Model file for the job. Use its own axes, mm. Face numbers are marked on the shaded views. Give positions to 0.01 mm unless a question says otherwise; leave off trailing zeros. Write each loop counter-clockwise with the first axis right and the second up, starting at its lowest first coordinate (ties: lowest second). Pieces come first, ordered by that corner, then holes.
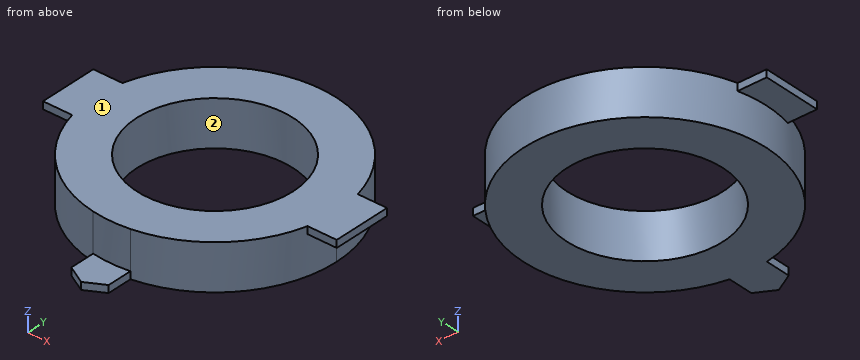
```python
from build123d import *

# Parameters (mm, degrees)
F1_DEPTH = 6.24
F2_DEPTH = 1
F3_R     = 10.71
F4_DEPTH = 6.241
F6_DEPTH = 1


# Not quite as in the source:
# - a pattern or mirror of a feature is missing from the dataset's text; its kind, count and spacing are read off the source's solid


with BuildPart() as f1:
    # F0 (on Top) → F1 (new body)
    with BuildSketch(Plane.XY):
        with BuildLine():
            ThreePointArc((2.56, -16.4317771407), (12.6318981155, -10.8162863313), (16.63, 0))
            ThreePointArc((16.63, 0), (-10.8162863313, 12.6318981155), (-2.56, -16.4317771407))
            ThreePointArc((-2.56, -16.4317771407), (0, -16.63), (2.56, -16.4317771407))
        make_face()
    extrude(amount=F1_DEPTH)

    # F0 (on Top) → F2 (join)
    with BuildSketch(Plane.XY):
        with BuildLine():
            ThreePointArc((2.56, -16.4317771407), (0, -16.63), (-2.56, -16.4317771407))
            Line((-2.56, -16.4317771407), (-2.56, -19.8917771407))
            Line((-2.56, -19.8917771407), (0, -21.31))
            Line((0, -21.31), (2.56, -19.8917771407))
            Line((2.56, -19.8917771407), (2.56, -16.4317771407))
        make_face()
    extrude(amount=F2_DEPTH)

    # F3 (on face) → F4 (cut, through all)
    with BuildSketch(Plane.XY.offset(6.24)):
        Circle(F3_R)
    extrude(amount=-F4_DEPTH, mode=Mode.SUBTRACT)

    # F5 (on face) → F6 (join)
    with BuildSketch(Plane.XY.offset(6.24)):
        with BuildLine():
            Line((20.1417749953, 4), (16.1417749953, 4))
            ThreePointArc((16.1417749953, 4), (16.5074925136, 2.0148426524), (16.63, 0))
            ThreePointArc((16.63, 0), (16.5074925136, -2.0148426524), (16.1417749953, -4))
            Line((16.1417749953, -4), (20.1417749953, -4))
            Line((20.1417749953, -4), (20.1417749953, 4))
        make_face()
    f6 = extrude(amount=-F6_DEPTH)

    # F6_copies: F6 across plane
    add(f6.mirror(Plane(origin=(0, 0, 0), x_dir=(0, 0, -1), z_dir=(-1, 0, 0))))


solid = f1.part
```
1. Slice it at D-D, the plane z = 3. Write the cut outline in (x, y), and give its area (3 significant figures).
Calculated:
outline: circle Ø33.26 at (0, 0); hole circle Ø21.42 at (0, 0)
area: 508 mm2
2. Pin check, flat tips, straight feed: P1, Ø1.2, axis at x = 18, y = -1, coming from the -Z side; P2, Ø0.5, axis at x = -17.5, z = 5.5, coming from the -Y side; P3, Ø1.1, axis at x = 18.5, z = 5.5, coming from the +Y side. Stop position of each tip, or through.
Calculated:
P1: stops at z = 5.24
P2: stops at y = -4
P3: stops at y = 4
3. Probe probe 1 along Y at (x, z) = (0, 4.5); probe 2 along X at (y, z) = (-7, 2.5); probe 3 along X at (y, z) = (3, 2). List the from-to ranges inside material, lowest first.
Calculated:
probe 1: y = -16.63 to -10.71, 10.71 to 16.63
probe 2: x = -15.08 to -8.11, 8.11 to 15.08
probe 3: x = -16.36 to -10.28, 10.28 to 16.36
4. Slice it at B-B, the plane z = 0.5. Write the cut outline in (x, y), and give its area (3 significant figures).
Calculated:
outline: (-2.56, -19.89) - (0, -21.31) - (2.56, -19.89) - (2.56, -16.43) arc R16.63 ccw (long way) to (-2.56, -16.43) - close; hole circle Ø21.42 at (0, 0)
area: 529 mm2
5. Pull direction Y, two halves, no side cores. Call the marked faces 1 and 2: +Y half, -Y half, draft (parallel to the pull), parting line (faces both ways), or undercut.
Calculated:
face 1: draft
face 2: undercut
6. Slice it at A-A, the plane y = -3. Write the cut outline in (x, z).
Calculated:
outline: (-20.14, 5.24) - (-16.36, 5.24) - (-16.36, 0) - (-10.28, 0) - (-10.28, 6.24) - (-20.14, 6.24) - close; (10.28, 0) - (16.36, 0) - (16.36, 5.24) - (20.14, 5.24) - (20.14, 6.24) - (10.28, 6.24) - close
7. Slice it at C-C, the plane y = 5.5. Write the cut outline in (x, z).
Calculated:
outline: (-15.69, 0) - (-9.19, 0) - (-9.19, 6.24) - (-15.69, 6.24) - close; (9.19, 0) - (15.69, 0) - (15.69, 6.24) - (9.19, 6.24) - close
